Design review of the part built by this model. Coordinates are the model's own, in mm. Face numbers are marked on the shaded views. A direction names the side the tool comes from. Coordinates: 2 decimals unless noted, no trailing zeros. Write each loop counter-clockwise with the first axis right and the second up, starting at its lowest first coordinate (ties: lowest second). Pieces come first, ordered by that corner, then holes. Notation, with made-up numbers: (31, 86) -> (70, 86) arc R15 ccw to (70, 92) -> close; hole circle Ø5 at (-5.75, 46.5). An arc over 180 degrees is marked (long way). Answer in a Markdown table with one row per item. Add a question column.
Item 1: To check wall thickness, follow line 1 (X direction, y = -0.65, z = 1.75) (3 decimals); line 2 (Z direction, x = -1.5, y = 2.1); line 3 (Z direction, x = -0.75, y = 1.2). State the ranges of each line that lie inside material, in increasing order.
Item 2: Take a section at C-C, the plane x = -2. Write out the cut boundary in (y, z).
Item 3: Clearance check with flat-ended pins moving along their axes: P1, Ø2, axis at x = -6, y = -0.5, coming from the +Z side; P2, Ø1.4, axis at x = -5.5, y = 0, coming from the -Z side; P3, Ø1.5, axis at y = 1.5, z = 4, coming from the -X side. State where each tip first meets the part, or that it passes through.
Item 4: Take a section at B-B, the plane x = 0.5. Write out the cut boundary in (y, z), and give its area (3 significant figures).
Item 5: For the marked faces 4, 5, 6 and 7, list the 3-axis set-ups (+Z, -Z, +X, -X, +Y, -Y) from which the entire face can be reached by the end or side of a thin tool; tool diameter is ignored.
Item 6: Draft analysis for pull direction Y (two halves, no side actions). For the marked faces 1, 2 and 3, state which applies: released by +Y, released by -Y, zero draft, split by the parting line, or undercut.
Item 7: Take a section at A-A, the plane x = -5.4. Write out the cut boundary in (y, z) (3 decimals), and give its area (3 significant figures).
from build123d import *

# Parameters (mm, degrees)
PAD_DEPTH    = 2.3
SKETCH001_R  = 0.635
PAD001_DEPTH = 1.6
SKETCH002_R  = 1.5
PAD002_DEPTH = 2.5
FILLET_R     = 1.45
CHAMFER_SIZE = 0.25


with BuildPart() as part:
    # Sketch → Pad (new body, symmetric)
    with BuildSketch(Plane.XZ):
        Polygon((-6.5, 0), (-4.765, 0), (-4.765, 1.8), (-1.265, 1.8), (-1.265, 0), (0, 0), (0, 5.3), (-1.71, 5.3), (-4.5, 2.51), (-6.5, 2.51), align=None)
    extrude(amount=PAD_DEPTH, both=True)

    # Sketch001 → Pad001 (join)
    with BuildSketch(Plane(origin=(0, 0, 0), x_dir=(-1, 0, 0), z_dir=(0, 0, -1))):
        with Locations((5.4, 1.27)):
            Circle(SKETCH001_R)
        with Locations((5.4, -1.27)):
            Circle(SKETCH001_R)
    extrude(amount=PAD001_DEPTH)

    # Sketch002 → Pad002 (join)
    with BuildSketch(Plane.YZ):
        with Locations((0, 3.75)):
            Circle(SKETCH002_R)
    extrude(amount=PAD002_DEPTH)

    # Fillet
    fillet_edges = [part.edges().sort_by_distance(p)[0] for p in [
        (2.5, -1.5, 3.75),
    ]]
    fillet(fillet_edges, radius=FILLET_R)

    # Chamfer
    chamfer_edges = [part.edges().sort_by_distance(p)[0] for p in [
        (-4.765, 1.27, -1.6),
        (-4.765, -1.27, -1.6),
    ]]
    chamfer(chamfer_edges, length=CHAMFER_SIZE)


solid = part.part
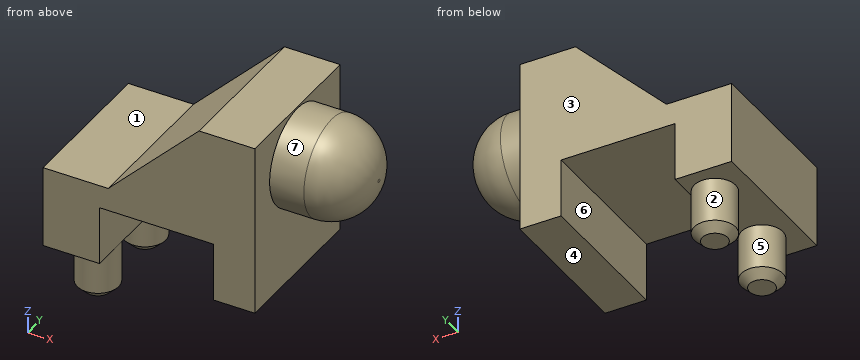
Answers:
| question | item | result |
|---|---|---|
| 1 | line 1 | x = -6.5 to -4.765, -1.265 to 0 |
| 1 | line 2 | z = 1.8 to 5.3 |
| 1 | line 3 | z = 0 to 5.3 |
| 2 | outline | (-2.3, 1.8) -> (2.3, 1.8) -> (2.3, 5.01) -> (-2.3, 5.01) -> close |
| 3 | P1 | stops at z = 2.51 |
| 3 | P2 | stops at z = -1.41 |
| 3 | P3 | stops at x = -3.76 |
| 4 | outline | circle Ø3 at (0, 3.75) |
| 4 | area | 7.07 mm^2 |
| 5 | face 4 | -Z, +X, +Y, -Y |
| 5 | face 5 | -Z |
| 5 | face 6 | -Z, +Y, -Y |
| 5 | face 7 | +X |
| 6 | face 1 | zero draft |
| 6 | face 2 | undercut |
| 6 | face 3 | released by +Y |
| 7 | outline | (-2.3, 0) -> (-1.905, 0) -> (-1.905, -1.35) -> (-1.655, -1.6) -> (-0.885, -1.6) -> (-0.635, -1.35) -> (-0.635, 0) -> (0.635, 0) -> (0.635, -1.35) -> (0.885, -1.6) -> (1.655, -1.6) -> (1.905, -1.35) -> (1.905, 0) -> (2.3, 0) -> (2.3, 2.51) -> (-2.3, 2.51) -> close |
| 7 | area | 15.5 mm^2 |
